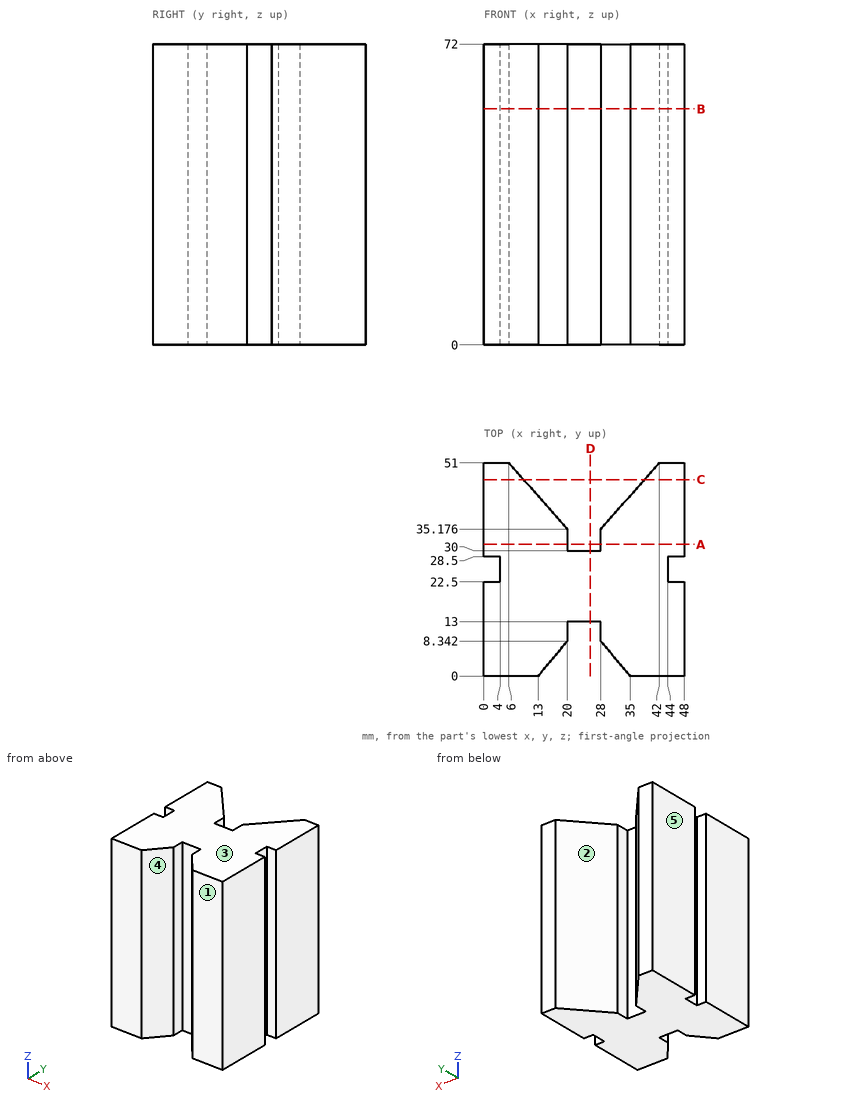
Print and shaded views of the part. All mm, measured from the part's lowest x, y and z. A direction names the side the tool comes from. Round coordinates to 2 decimals unless told otherwise and drop trailing zeros. Write each loop counter-clockwise with the first axis right and the second up, starting at its lowest first coordinate (ties: lowest second). Pieces come first, ordered by that corner, then holes. Notation, with made-up numbers: M 85.5,87.5 L 93.5,87.5 A21 cw 93.5,102.5 Z; hole C 24,50 d11. An arc over 180 degrees is marked long. Use a Markdown table: item, result. Add a question column.
1. Slice it at A-A on y = 31.5. Give the cut face in (x, z).
2. Slice it at C-C on y = 47. Give the cut face in (x, z).
3. 3-axis set-ups, long thin cutter, end or side, ignore diameter. For the marked faces 1 and 2: which of +Z, -Z, +X, -X, +Y, -Y reach the whole face in a straight line?
4. Pull direction X, two halves, no side cores. Call the marked faces 3, 4 and 5: released by +X, released by -X, zero draft, split by the parting line, or undercut.
5. Drill centre lines: probe 1 along X at (y, z) = (11.5, 6.5); probe 2 along Y at (x, z) = (22, 10.5); probe 3 along X at (y, z) = (42, 7.5). Where is each one in solid material? Low to high.
6. Flat gauge pins, fed straight in: P1, Ø12, axis at x = 21.5, z = 60, coming from the -Y side; P2, Ø6.5, axis at x = 24.5, z = 51.5, coming from the +Y side; P3, Ø1.8, axis at y = 24.5, z = 36.5, coming from the -X side; P4, Ø1.6, axis at y = 32, z = 48.5, coming from the -X side. Where does each tip first touch, or does it go through?
7. Slice it at B-B on z = 56.5. Give the cut face in (x, y), then the cut area to 3 significant figures.
8. Slice it at D-D on x = 25.5. Give the cut face in (y, z).
Reply:
| question | item | result |
|---|---|---|
| 1 | outline | M 0,0 L 20,0 L 20,72 L 0,72 Z; M 28,0 L 48,0 L 48,72 L 28,72 Z |
| 2 | outline | M 0,0 L 9.54,0 L 9.54,72 L 0,72 Z; M 38.46,0 L 48,0 L 48,72 L 38.46,72 Z |
| 3 | face 1 | +Z, -Z, +X, -X, -Y |
| 3 | face 2 | +Z, -Z, +Y |
| 4 | face 3 | zero draft |
| 4 | face 4 | undercut |
| 4 | face 5 | released by -X |
| 5 | probe 1 | x = 0 to 20, 28 to 48 |
| 5 | probe 2 | y = 13 to 30 |
| 5 | probe 3 | x = 0 to 13.96, 34.04 to 48 |
| 6 | P1 | stops at y = 2.98 |
| 6 | P2 | stops at y = 30 |
| 6 | P3 | stops at x = 4 |
| 6 | P4 | stops at x = 0 |
| 7 | outline | M 0,0 L 13,0 L 20,8.34 L 20,13 L 28,13 L 28,8.34 L 35,0 L 48,0 L 48,22.5 L 44,22.5 L 44,28.5 L 48,28.5 L 48,51 L 42,51 L 28,35.18 L 28,30 L 20,30 L 20,35.18 L 6,51 L 0,51 L 0,28.5 L 4,28.5 L 4,22.5 L 0,22.5 Z |
| 7 | area | 1,850 mm^2 |
| 8 | outline | M 13,0 L 30,0 L 30,72 L 13,72 Z |
